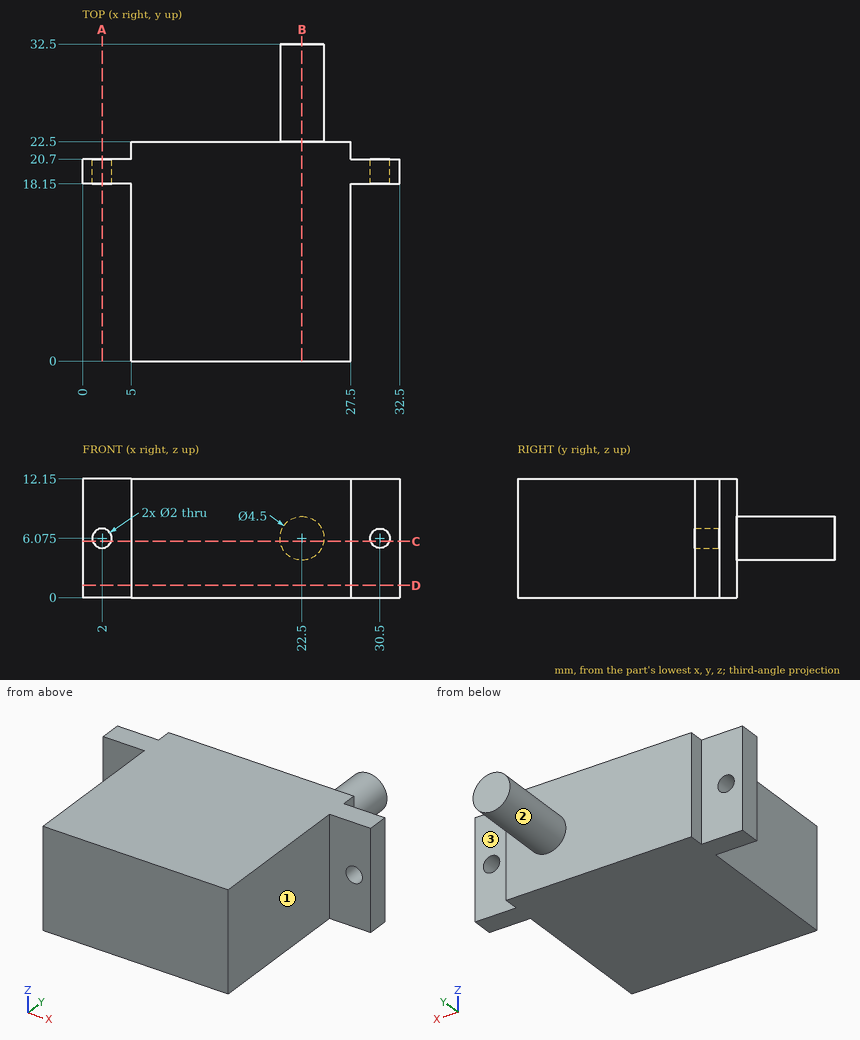
Verification items for this drawing (mm, ordinates from the low corner). A direction names the side the tool comes from. Coordinates: 2 decimals unless noted, no trailing zeros. Write each loop counter-clockwise with the first axis right and the second up, starting at its lowest first coordinate (ties: lowest second). Pieces come first, ordered by that corner, then holes. Notation, with made-up numbers: (69.5, 14.25) -> (95.5, 14.25) arc R16 cw to (95.5, 29.25) -> close; hole circle Ø3 at (-33, 48.5). An arc over 180 degrees is marked (long way). Use CSV: the item, a comma, the result in double quotes. Start each with the question number.
Item 1: Set-up check for the marked faces 1, 2 and 3: record each of +Z, -Z, +X, -X, +Y, -Y from which the full face is reachable in a straight line by a thin tool's end or side.
Item 2: Cross-section at C-C, the plane z = 5.75. Record the cut outline in (x, y), plus the area to 3 significant figures.
Item 3: Depth check by flat-ended pin: pin 1 Ø3 at (x, z) = (2, 6.075) entering from +Y; pin 2 Ø1 at (y, z) = (7, 7) entering from -X; pin 3 Ø5.5 at (x, z) = (30.5, 4.5) entering from -Y. Enter the tip coordinate at first touch or a pass-through.
Item 4: Cross-section at D-D, the plane z = 1.25. Record the cut outline in (x, y).
Item 5: Cross-section at B-B, the plane x = 22.5. Record the cut outline in (y, z) (3 decimals), plus the area to 3 significant figures.
Item 6: Thickness scan on line 1 (Y direction, x = 14, z = 8.25); line 2 (X direction, y = 7, z = 10.5); line 3 (Z direction, x = 30, y = 19). Record the ranges inside material, lowest first.
Item 7: Cross-section at A-A, the plane x = 2. Record the cut outline in (y, z) (3 decimals).
Answers:
1,face 1,"+Z, -Z, +X, -Y"
1,face 2,"+Y"
1,face 3,"+Z, -Z, +X, +Y"
2,outline,"(0, 18.15) -> (1.05, 18.15) -> (1.05, 20.7) -> (0, 20.7) -> close; (2.95, 18.15) -> (5, 18.15) -> (5, 0) -> (27.5, 0) -> (27.5, 18.15) -> (29.55, 18.15) -> (29.55, 20.7) -> (27.5, 20.7) -> (27.5, 22.5) -> (24.73, 22.5) -> (24.73, 32.5) -> (20.27, 32.5) -> (20.27, 22.5) -> (5, 22.5) -> (5, 20.7) -> (2.95, 20.7) -> close; (31.45, 18.15) -> (32.5, 18.15) -> (32.5, 20.7) -> (31.45, 20.7) -> close"
2,area,"567 mm^2"
3,pin 1,"y = 20.7"
3,pin 2,"x = 5"
3,pin 3,"y = 18.15"
4,outline,"(0, 18.15) -> (5, 18.15) -> (5, 0) -> (27.5, 0) -> (27.5, 18.15) -> (32.5, 18.15) -> (32.5, 20.7) -> (27.5, 20.7) -> (27.5, 22.5) -> (5, 22.5) -> (5, 20.7) -> (0, 20.7) -> close"
5,outline,"(0, 0) -> (22.5, 0) -> (22.5, 3.825) -> (32.5, 3.825) -> (32.5, 8.325) -> (22.5, 8.325) -> (22.5, 12.15) -> (0, 12.15) -> close"
5,area,"318 mm^2"
6,line 1,"0 to 22.5"
6,line 2,"5 to 27.5"
6,line 3,"0 to 5.21, 6.94 to 12.15"
7,outline,"(18.15, 0) -> (20.7, 0) -> (20.7, 5.075) -> (18.15, 5.075) -> close; (18.15, 7.075) -> (20.7, 7.075) -> (20.7, 12.15) -> (18.15, 12.15) -> close"
